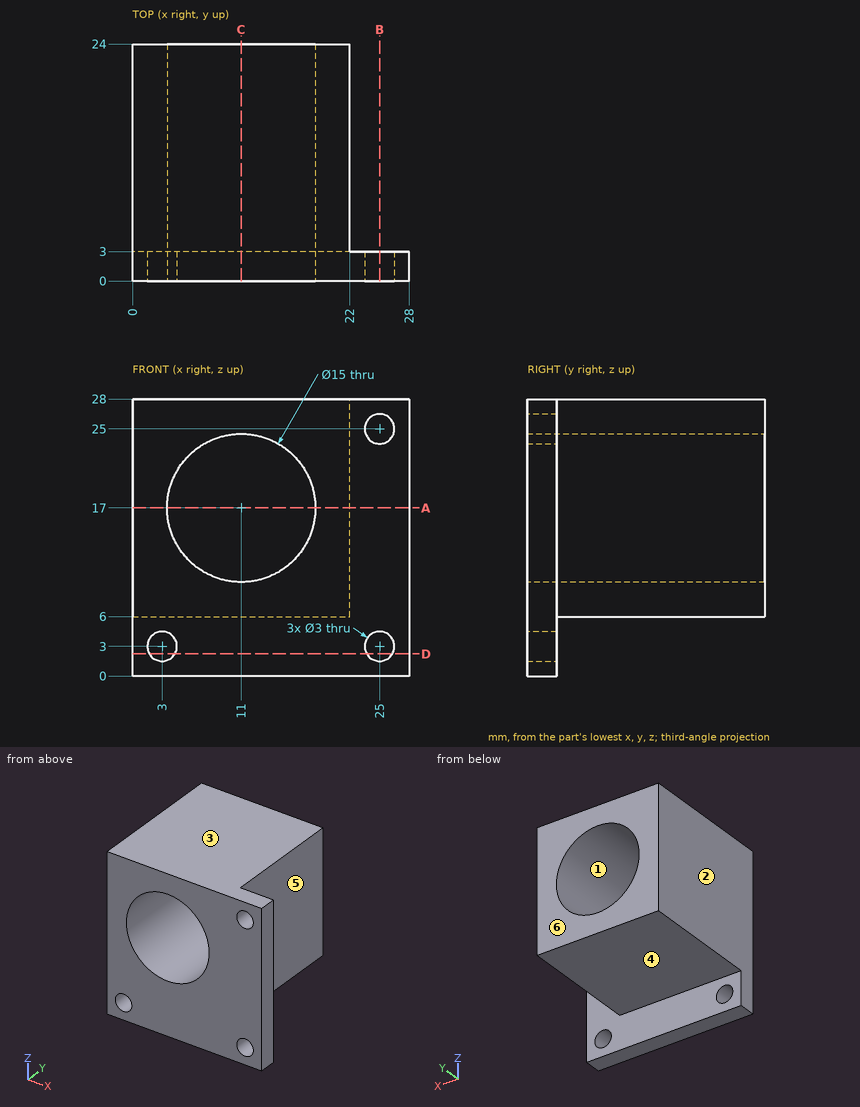
Geometry check sheet. Reference: drawing and pictorial views, mm from the part's lowest x, y, z. A direction names the side the tool comes from. Round coordinates to 2 decimals unless told otherwise and drop trailing zeros. Loops run counter-clockwise (first coordinate to the right, second up) from the corner with the lowest first, then second, coordinate; pieces in that order, holes last. Notation, with made-up numbers: (17.5, 41.5) -> (23.5, 41.5) arc R29 cw to (23.5, 68.5) -> close; hole circle Ø10 at (34, -31). An arc over 180 degrees is marked (long way). Answer as a JSON object with one key per item and string values.
Q1. Section check D-D (z = 2.25). Record the boundary of the cut face in (x, y).
Data:
{"outline": "(0, 0) -> (1.7, 0) -> (1.7, 3) -> (0, 3) -> close; (4.3, 0) -> (23.7, 0) -> (23.7, 3) -> (4.3, 3) -> close; (26.3, 0) -> (28, 0) -> (28, 3) -> (26.3, 3) -> close"}
Q2. Scan lines: line 1 (X direction, y = 2.15, z = 3); line 2 (Z direction, x = 11.25, y = 21); line 3 (X direction, y = 3.75, z = 25.25). Record each from-to range of solid material in increasing order. Write a range as from..to.
Data:
{"line 1": "x = 0..1.5, 4.5..23.5, 26.5..28", "line 2": "z = 6..9.5, 24.5..28", "line 3": "x = 0..22"}
Q3. Section check C-C (x = 11). Record the boundary of the cut face in (y, z), then the cut area to 3 significant figures.
Data:
{"outline": "(0, 0) -> (3, 0) -> (3, 6) -> (24, 6) -> (24, 9.5) -> (0, 9.5) -> close; (0, 24.5) -> (24, 24.5) -> (24, 28) -> (0, 28) -> close", "area": "186 mm2"}
Q4. Draft check along Z on the marked faces 1, 2 and 3. Enter one of: pulls with the +Z half, pulls with the -Z half, needs draft (parallel to the pull), parting line crosses it, or undercut.
Data:
{"face 1": "undercut", "face 2": "needs draft", "face 3": "pulls with the +Z half"}
Q5. Section check B-B (x = 25). Record the boundary of the cut face in (y, z), then the cut area to 3 significant figures.
Data:
{"outline": "(0, 0) -> (3, 0) -> (3, 1.5) -> (0, 1.5) -> close; (0, 4.5) -> (3, 4.5) -> (3, 23.5) -> (0, 23.5) -> close; (0, 26.5) -> (3, 26.5) -> (3, 28) -> (0, 28) -> close", "area": "66.0 mm2"}
Q6. Go/stop test with flat-tipped pins: P1, Ø8, axis at y = 12.5, z = 5, coming from the +X side; P2, Ø1.8, axis at x = 25, z = 25, coming from the +Y side; P3, Ø3.5, axis at x = 3, z = 3, coming from the +Y side. Record where each tip stops, or that it passes through.
Data:
{"P1": "stops at x = 22", "P2": "passes through", "P3": "stops at y = 3"}
Q7. Section check A-A (z = 17). Record the boundary of the cut face in (x, y).
Data:
{"outline": "(0, 0) -> (3.5, 0) -> (3.5, 24) -> (0, 24) -> close; (18.5, 0) -> (28, 0) -> (28, 3) -> (22, 3) -> (22, 24) -> (18.5, 24) -> close"}
Q8. Access from +Z, -Z, +X, -X, +Y, -Y to the whole of each face (thin tool, end or side, straight path). Record for the marked faces 4, 5 and 6.
Data:
{"face 4": "-Z, +X, -X, +Y", "face 5": "+Z, -Z, +X, +Y", "face 6": "+Z, -Z, +X, -X, +Y"}
